from build123d import *

# Parameters (mm, degrees)
M8_CLEARANCE_HOLE1_D     = 9
M8_CLEARANCE_HOLE1_DEPTH = 15
CIRPATTERN1_COUNT        = 5


with BuildPart() as part:
    # Sketch2 → Revolve1 (revolve)
    with BuildSketch(Plane.XY):
        Polygon((-30, 9), (0, 9), (0, 17.5), (-15, 17.5), (-15, 60), (-30, 60), (-30, 37.5), (-20, 37.5), (-20, 12.5), (-30, 12.5), align=None)
    revolve(axis=Axis((-30, 0, 0), (1, 0, 0)))

    # M8 Clearance Hole1
    with Locations(Plane(origin=(-15, -50, 0), x_dir=(0, 0, 1), z_dir=(1, 0, 0))):
        with Locations((0, 0)):
            m8_clearance_hole1 = Hole(M8_CLEARANCE_HOLE1_D / 2, depth=M8_CLEARANCE_HOLE1_DEPTH)

    # CirPattern1: M8 Clearance Hole1 ×5 about axis
    cirpattern1_axis = Axis((0, 0, 0), (1, 0, 0))
    for i in range(1, CIRPATTERN1_COUNT):
        add(m8_clearance_hole1.rotate(cirpattern1_axis, i * 360 / CIRPATTERN1_COUNT), mode=Mode.SUBTRACT)


solid = part.part
Check sheet for the modelled part. Datum: model origin and axes. Units: mm. A direction names the side the tool comes from. Round coordinates to 2 decimals unless told otherwise and drop trailing zeros. Order: outer loops, then holes, each group sorted by start corner. A loop starts at its lowest first (then second) coordinate and runs counter-clockwise, first axis right, second up.
Q1. Cross-section at C-C, the plane x = -23.5. Give the number of separate pieces and of enclosed holes in the cut face, plus the area to 3 significant figures.
Filled sheet:
separate pieces: 2
enclosed holes: 7
area: 6,810 mm2
Q2. Cross-section at B-B, the plane y = 0. Enter the section's corners in (x, z), plus the area to 4 significant figures.
Filled sheet:
outline: (-30, -60) - (-15, -60) - (-15, -17.5) - (0, -17.5) - (0, -9) - (-30, -9) - (-30, -12.5) - (-20, -12.5) - (-20, -37.5) - (-30, -37.5) - close; (-30, 9) - (0, 9) - (0, 17.5) - (-15, 17.5) - (-15, 60) - (-30, 60) - (-30, 37.5) - (-20, 37.5) - (-20, 12.5) - (-30, 12.5) - close
area: 1,285 mm2
Q3. Cross-section at D-D, the plane x = -11.5. Enter the section's corners in (y, z), plus the area to 3 significant figures.
Filled sheet:
outline: circle Ø35 at (0, 0); hole circle Ø18 at (0, 0)
area: 708 mm2
Q4. Set-up check for faces 4 (the face through (-22.6, -45.61, 0.98)), 5 (the face through (-20, -9, 9)): record each of +Z, -Z, +X, -X, +Y, -Y from which the full face is reachable in a straight line by a thin tool's end or side.
Filled sheet:
face 4: +X, -X
face 5: -X
Q5. Cross-section at A-A, the plane z = 0. Enter the section's corners in (x, y).
Filled sheet:
outline: (-30, -60) - (-15, -60) - (-15, -54.5) - (-30, -54.5) - close; (-30, -45.5) - (-15, -45.5) - (-15, -17.5) - (0, -17.5) - (0, -9) - (-30, -9) - (-30, -12.5) - (-20, -12.5) - (-20, -37.5) - (-30, -37.5) - close; (-30, 9) - (0, 9) - (0, 17.5) - (-15, 17.5) - (-15, 60) - (-30, 60) - (-30, 37.5) - (-20, 37.5) - (-20, 12.5) - (-30, 12.5) - close
Q6. Scan lines: L1, parallel to Z at x = -25, y = 0; L2, parallel to Y at x = -22, z = -33; L3, parallel to X at y = -23.5, z = -20. Record each from-to range of solid material in increasing order.
Filled sheet:
L1: z = -60 to -37.5, -12.5 to -9, 9 to 12.5, 37.5 to 60
L2: y = -50.11 to -17.81, 17.81 to 37.77, 43.14 to 50.11
L3: x = -20 to -15
Q7. Depth check by flat-ended pin: P1, Ø10, axis at x = -8.5, y = -2, coming from the +Z side; P2, Ø5, axis at x = -23, z = -13, coming from the -Y side; P3, Ø4, axis at y = -44.5, z = 24, coming from the +X side; P4, Ø7, axis at y = -50, z = 0, coming from the +X side. Enter the tip coordinate at first touch or a pass-through.
Filled sheet:
P1: stops at z = 17.5
P2: stops at y = -59.07
P3: stops at x = -15
P4: passes through
Q8. Draft check along Z on faces 1 (the face through (-7.605, -13.887, -10.648)), 2 (the face through (-15, -12.5, -12.5)), 3 (the face through (-24.93, -4.88, 37.18)). Enter one of: pulls with the +Z half, pulls with the -Z half, needs draft (parallel to the pull), parting line crosses it, or undercut.
Filled sheet:
face 1: parting line crosses it
face 2: needs draft
face 3: undercut
